Build history of the part. All positions in model axes, mm. Give positions to 0.01 mm unless a question says otherwise; leave off trailing zeros. Write each loop counter-clockwise with the first axis right and the second up, starting at its lowest first coordinate (ties: lowest second). Pieces come first, ordered by that corner, then holes.
Autodesk Inventor part; units mm, degrees
ref_plane "Work Plane2" through (0, 0, 2209) normal (0, 0, 1) x (1, 0, 0)
ref_plane "Work Plane3" through (0, -100, 0) normal (1, 0, 0) x (0, 1, 0)
ref_plane "YZ Plane" through (0, 0, 0) normal (1, 0, 0) x (0, 1, 0)
ref_plane "Work Plane2" through (0, 0, 2209) normal (0, 0, 1) x (1, 0, 0)
ref_plane "Work Plane1" through (0, 0, 0) normal (0, 0, 1) x (1, 0, 0)
sketch "Sketch1" plane through (0, 0, 0) normal (0, 0, 1) x (1, 0, 0)
  line L0 (0, 0) -> (1369, 0)
  line L1 (1369, 0) -> (1369, -100)
  line L2 (1369, -100) -> (0, -100)
  line L3 (0, -100) -> (0, 0)
  dimension "d2" = 1369
  dimension "d3" = 100
sketch "Sketch2" plane through (0, 0, 2209) normal (0, 0, 1) x (1, 0, 0)
  line L0 (0, -100) -> (0, 0)
  line L1 (1369, 0) -> (1369, -100)
ref_plane "Work Plane3" through (0, -100, 0) normal (1, 0, 0) x (0, 1, 0)
sketch "Sketch3" plane through (0, -100, 0) normal (1, 0, 0) x (0, 1, 0)
  line L0 (0, 2209) -> (100, 2209)
  line L1 (0, 0) -> (100, 0) construction
  line L2 (100, 0) -> (-289.5063, 2209)
  line L3 (100, 0) -> (2343.0774, 0) construction
  line L4 (-289.5063, 2209) -> (-389.5063, 2209)
  line L5 (-389.5063, 2209) -> (0, 0)
  dimension "d4" = 100
  dimension "d5" = 100
sketch "Sketch4" plane through (0, 0, 2209) normal (0, 0, 1) x (1, 0, 0)
  line L0 (0, -389.5063) -> (0, -489.5063)
  line L1 (1369, 0) -> (1369, -100)
  line L2 (0, -389.5063) -> (1369, -389.5063)
  line L3 (1369, -389.5063) -> (1369, -489.5063)
  line L4 (1369, -489.5063) -> (0, -489.5063)
  line L5 (0, -489.5063) -> (0, -389.5063)
  point P0 (0, 0)
loft "Loft1" add profiles "Sketch1", "Sketch4"
sketch "Sketch5" plane through (1369, -100, 0) normal (1, 0, 0) x (0, 0, -1)
  line L0 (0, 100) -> (0, 0)
  line L1 (0, 100) -> (-2209, -289.5063)
  line L2 (-2209, -289.5063) -> (-2209, -389.5063)
  line L3 (0, 0) -> (-2209, -389.5063)
  line L4 (-2209, -289.5063) -> (-1864.3173, -228.7294)
  line L5 (0, 100) -> (-2209, -289.5063)
  line L6 (-1864.3173, -228.7294) -> (-1864.3173, -238.7294)
  line L7 (-1864.3173, -238.7294) -> (-1844.6211, -235.2565)
  line L8 (-1844.6211, -235.2565) -> (-1844.6211, -225.2565)
  line L9 (-1844.6211, -225.2565) -> (-1499.9384, -164.4796)
  line L10 (-1499.9384, -164.4796) -> (-1499.9384, -174.4796)
  line L11 (-1499.9384, -174.4796) -> (-1480.2423, -171.0066)
  line L12 (-1480.2423, -171.0066) -> (-1480.2423, -161.0066)
  line L13 (-1480.2423, -161.0066) -> (-1135.5595, -100.2298)
  line L14 (-1135.5595, -100.2298) -> (-1135.5595, -110.2298)
  line L15 (-1135.5595, -110.2298) -> (-1116.23, -106.8215)
  line L16 (-1116.23, -106.8215) -> (-1116.23, -96.8215)
  line L17 (-1116.23, -96.8215) -> (-771.5473, -36.0446)
  line L18 (-771.5473, -36.0446) -> (-771.5473, -46.0446)
  line L19 (-771.5473, -46.0446) -> (-752.0292, -42.603)
  line L20 (-752.0292, -42.603) -> (-752.0292, -32.603)
  line L21 (-752.0292, -32.603) -> (-407.3465, 28.1738)
  line L22 (-407.3465, 28.1738) -> (-407.3465, 18.1738)
  line L23 (-407.3465, 18.1738) -> (-387.7831, 21.6234)
  line L24 (-387.7831, 21.6234) -> (-387.7831, 31.6234)
  line L25 (-387.7831, 31.6234) -> (0, 100)
  line L26 (-387.7831, 31.6234) -> (-1864.3173, -228.7294)
  point P0 (-771.5473, -36.0446)
  point P1 (-1135.5595, -100.2298)
  dimension "d10" = 350
  dimension "d11" = 10
  dimension "d12" = 20
  dimension "d13" = 350
  dimension "d14" = 20
  dimension "d15" = 350
  dimension "d16" = 350
  dimension "d17" = 350
extrude "Extrusion1" cut sketch "Sketch5" against normal through all contours L24 L23 L22 L1 | L20 L19 L18 L1 | L1 L8 L7 L6 | L16 L15 L14 L1 | L1 L12 L11 L10
properties part number "eave_panel_01" material "Wood (Maple)"
1. Drop a flat-ended pin along its axis: pin 1 (3 mm diameter, centred on x = 1157, z = 787.5, fed in from +Y). Give the stop position or say it passes through.
2. Drill centre lines: line 1 along Y through (x, z) = (479.5, 2044.5); line 2 along Y through (x, z) = (1140, 1984). Where is each one in solid material? Low to high.
3. Saw through at A-A on x = 1218. Give the cut face in (y, z), plus the area to 3 significant figures.
Outcome:
1. pin 1: stops at y = -138.59
2. line 1: y = -460.5 to -360.5
2. line 2: y = -449.83 to -349.83
3. outline: (-489.51, 2209) - (-100, 0) - (0, 0) - (-68.38, 387.78) - (-78.38, 387.78) - (-81.83, 407.35) - (-71.83, 407.35) - (-132.6, 752.03) - (-142.6, 752.03) - (-146.04, 771.55) - (-136.04, 771.55) - (-196.82, 1116.23) - (-206.82, 1116.23) - (-210.23, 1135.56) - (-200.23, 1135.56) - (-261.01, 1480.24) - (-271.01, 1480.24) - (-274.48, 1499.94) - (-264.48, 1499.94) - (-325.26, 1844.62) - (-335.26, 1844.62) - (-338.73, 1864.32) - (-328.73, 1864.32) - (-389.51, 2209) - close
3. area: 220,000 mm2
